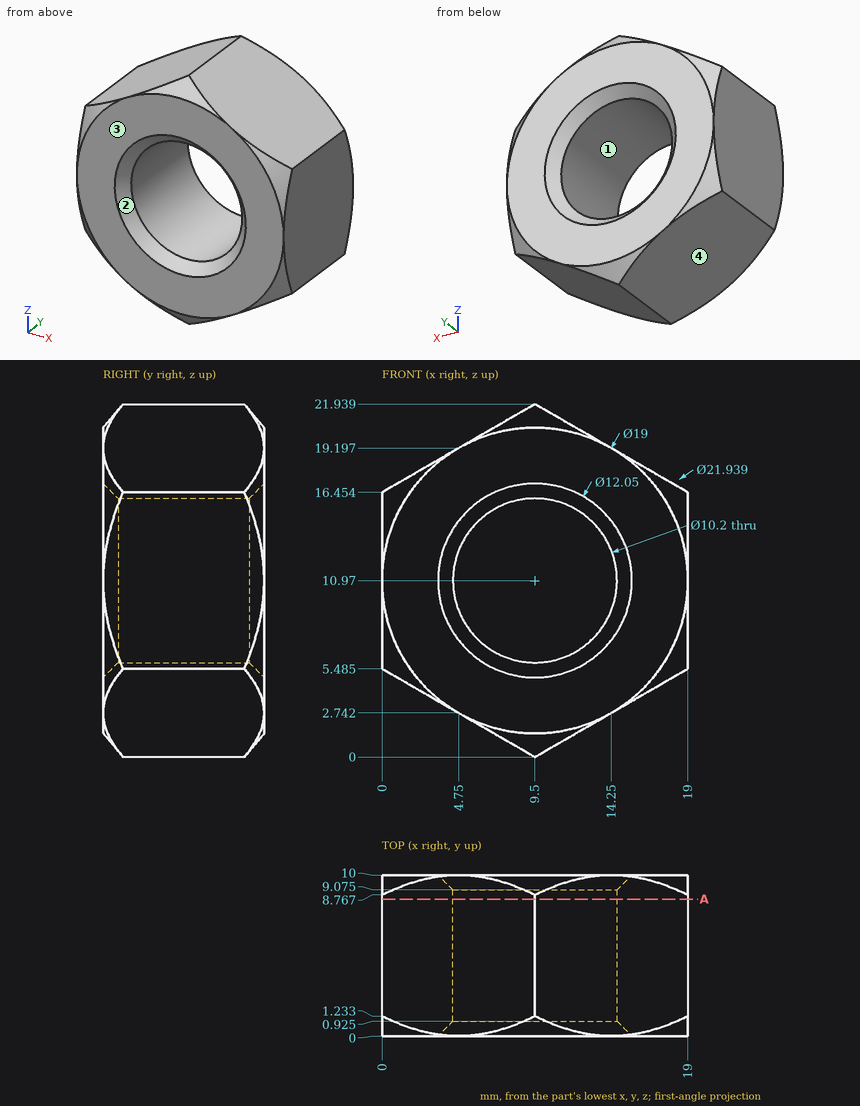
Verification items for this drawing (mm, ordinates from the low corner). Give positions to 0.01 mm unless a question says otherwise; leave off trailing zeros. Loops run counter-clockwise (first coordinate to the right, second up) from the corner with the lowest first, then second, coordinate; pieces in that order, holes last. Notation, with made-up numbers: M -16,48 L 12,48 A24 ccw 12,74 Z; hole C 77.25,85.5 d4. An arc over 180 degrees is marked long. Write item = value, one per line. Start each with the question number.
1. Section check A-A, the plane y = 8.5. Enter the section's corners in (x, z) (1 decimal).
2. Thickness scan on probe 1 along Z at (x, y) = (14, 3) (1 decimal); probe 2 along X at (y, z) = (2, 14.75) (1 decimal); probe 3 along X at (y, z) = (5.5, 8) (1 decimal). Record the ranges inside material, lowest first.
3. Go/stop test with flat-tipped pins: P1, Ø1, axis at y = 8.5, z = 17.5, coming from the +X side (1 decimal); P2, Ø4, axis at x = 12, y = 5, coming from the -Z side; P3, Ø2, axis at x = 8, y = 3, coming from the +Z side. Record where each tip stops, or that it passes through.
4. Draft check along X on the marked faces 1, 2, 3 and 4. Enter one of: +X half, -X half, draft (parallel to the pull), parting line (faces both ways), or undercut.
Values follow:
q1.outline = M 0,5.5 L 9.5,0 L 19,5.5 L 19,16.5 L 9.5,21.9 L 0,16.5 Z; hole C 9.5,11 d10.2
q2.probe_1 = 2.6 to 8.6, 13.4 to 19.3
q2.probe_2 = 0 to 6.1, 12.9 to 19
q2.probe_3 = 0 to 5.4, 13.6 to 19
q3.P1 = 18.1
q3.P2 = 0.29
q3.P3 = 21.65
q4.face_1 = undercut
q4.face_2 = undercut
q4.face_3 = draft
q4.face_4 = -X half
